Check sheet for the modelled part. Datum: model origin and axes. Units: mm. A direction names the side the tool comes from. Round coordinates to 2 decimals unless told otherwise and drop trailing zeros. Order: outer loops, then holes, each group sorted by start corner. A loop starts at its lowest first (then second) coordinate and runs counter-clockwise, first axis right, second up. Notation, with made-up numbers: (-16, -33) -> (34, -33) arc R22 cw to (34, -10) -> close; hole circle Ø11 at (88.5, -37). An arc over 180 degrees is marked (long way). Use CSV: the item, a comma, the result in double quotes.
```python
from build123d import *

# Parameters (mm, degrees)
F0_W     = 120.6107288599
F0_H     = 61.03855744
F1_DEPTH = 76.2
F3_ANGLE = 180
F4_W     = 120.6107288599
F4_H     = 13.4453041246
F5_DEPTH = 25.4
F6_R     = 1.27
F7_R     = 4.935476451
F8_DEPTH = 76.2


with BuildPart() as f1:
    # F0 (on Front) → F1 (new body)
    with BuildSketch(Plane.XZ):
        Rectangle(F0_W, F0_H)
    extrude(amount=F1_DEPTH)

    # F2 (on face) → F3 (revolve, cut)
    with BuildSketch(Plane.XY.offset(30.51927872)):
        Polygon((0, -76.2), (0, 0), (-13.3808227256, 0), (-13.3808227256, -41.6820123792), (-22.573298703, -41.6820123792), (-25.4785586149, -28.1363911927), (-30.1583929265, -41.6820123792), (-38.8593822718, -41.6820123792), (-38.8593822718, -76.2), align=None)
    revolve(axis=Axis((0, -30.7025797665, 30.51927872), (0, -1, 0)), revolution_arc=F3_ANGLE, mode=Mode.SUBTRACT)

    # F4 (on face) → F5 (cut)
    with BuildSketch(Plane.XZ.offset(76.2)):
        with Locations((0, 5.0255007227)):
            Rectangle(F4_W, F4_H)
    extrude(amount=-F5_DEPTH, mode=Mode.SUBTRACT)

    # F6
    f6_edges = [f1.edges().sort_by_distance(p)[0] for p in [
        (0, -28.136391, 5.04072),
    ]]
    fillet(f6_edges, radius=F6_R)

    # F7 (on face) → F8 (cut)
    with BuildSketch(Plane.XZ.offset(76.2)):
        with Locations((-44.7249487042, -16.4052583277)):
            Circle(F7_R)
        with Locations((44.7249487042, -16.4052583277)):
            Circle(F7_R)
    extrude(amount=-F8_DEPTH, mode=Mode.SUBTRACT)


solid = f1.part
```
Q1. Sectioned sample at B-B, the plane z = -18. Enter the section's corners in (x, y), then the cut area to 3 significant figures.
Result sheet:
outline,"(-60.31, -76.2) -> (-49.4, -76.2) -> (-49.4, 0) -> (-60.31, 0) -> close; (-40.05, -76.2) -> (40.05, -76.2) -> (40.05, 0) -> (-40.05, 0) -> close; (49.4, -76.2) -> (60.31, -76.2) -> (60.31, 0) -> (49.4, 0) -> close"
area,"7,770 mm^2"
Q2. Mould release check, pull along X, two halves, no side actions. Record for faces 6 (the face through (60.305, -38, 0)), 7 (the face through (45, -50.8, 5)), 8 (the face through (-0.605, -34.046, 3.006)), 9 (the face through (-0.29, -21.13, 17.14)): pulls with the +X half, pulls with the -X half, needs draft (parallel to the pull), parting line crosses it, or undercut.
Result sheet:
face 6,"pulls with the +X half"
face 7,"needs draft"
face 8,"undercut"
face 9,"undercut"
Q3. Sectioned sample at D-D, the plane y = -13. Enter the section's corners in (x, z).
Result sheet:
outline,"(-60.31, -30.52) -> (60.31, -30.52) -> (60.31, 30.52) -> (13.38, 30.52) arc R13.38 cw to (-13.38, 30.52) -> (-60.31, 30.52) -> close; hole circle Ø9.87 at (-44.72, -16.41); hole circle Ø9.87 at (44.72, -16.41)"
Q4. Go/stop test with flat-tipped pins: pin 1 (6 mm diameter, centred on x = 44.72, z = -16.41, fed in from +Y); pin 2 (11.5 mm diameter, centred on x = 16.5, z = 4, fed in from -Y); pin 3 (4 mm diameter, centred on x = 34.5, z = 8, fed in from -Y). Record where each tip stops, or that it passes through.
Result sheet:
pin 1,"passes through"
pin 2,"stops at y = -41.68"
pin 3,"stops at y = -50.8"
Q5. Access from +Z, -Z, +X, -X, +Y, -Y to the whole of each face (thin tool, end or side, straight path). Record for faces 1 (the face through (47, -64, 11.748)), 2 (the face through (0, -41.682, -1)), 3 (the face through (-60.305, -38, 0)), 4 (the face through (-0.509, -39.093, 7.396)), 5 (the face through (-47, -76.2, 21)).
Result sheet:
face 1,"+X, -X, -Y"
face 2,"+Z, -Y"
face 3,"+Z, -Z, -X, +Y, -Y"
face 4,"-Y"
face 5,"+Z, -Z, +X, -X, -Y"
Q6. Sectioned sample at A-A, the plane y = -69. Enter the section's corners in (x, z), then the cut area to 3 significant figures.
Result sheet:
outline,"(-60.31, -30.52) -> (60.31, -30.52) -> (60.31, -1.7) -> (21.73, -1.7) arc R38.86 cw to (-21.73, -1.7) -> (-60.31, -1.7) -> close; (-60.31, 11.75) -> (-34.02, 11.75) arc R38.86 cw to (-38.86, 30.52) -> (-60.31, 30.52) -> close; (34.02, 11.75) -> (60.31, 11.75) -> (60.31, 30.52) -> (38.86, 30.52) arc R38.86 cw to start; hole circle Ø9.87 at (-44.72, -16.41); hole circle Ø9.87 at (44.72, -16.41)"
area,"3,990 mm^2"
Q7. Scan lines: L1, parallel to Z at x = 45, y = -5.5; L2, parallel to X at y = -10, z = -16; L3, parallel to X at y = -45, z = 6. Record each from-to range of solid material in increasing order.
Result sheet:
L1,"z = -30.52 to -21.33, -11.48 to 30.52"
L2,"x = -60.31 to -49.64, -39.81 to 39.81, 49.64 to 60.31"
L3,"x = -60.31 to -30.15, 30.15 to 60.31"
Q8. Sectioned sample at C-C, the plane x = -31.5. Enter the section's corners in (y, z).
Result sheet:
outline,"(-76.2, -30.52) -> (0, -30.52) -> (0, 30.52) -> (-41.68, 30.52) -> (-41.68, 7.76) -> (-50.8, 7.76) -> (-50.8, -1.7) -> (-76.2, -1.7) -> close"
